CAD build for the part. Positions are in the model's coordinates, mm. Face numbers are marked on the shaded views. A direction names the side the tool comes from. Coordinates: 2 decimals unless noted, no trailing zeros. Write each loop counter-clockwise with the first axis right and the second up, starting at its lowest first coordinate (ties: lowest second). Pieces come first, ordered by that corner, then holes. Notation, with made-up numbers: (49, 53) - (96, 53) arc R34 cw to (96, 87) - close; hole circle Ø10 at (12, 26). An arc over 180 degrees is marked (long way). One line per question, with ' | ' between items. Start each with the question number.
1. Band-saw the part on C-C, the plane x = 85. Write the cut outline in (y, z).
2. Probe line 1 (X direction, y = -0.5, z = 56.5); line 2 (Z direction, x = 64, y = 27); line 3 (X direction, y = -10, z = 79). List the from-to ranges inside material, lowest first.
3. Two-plate mould, pull along X, no slides. Class the marked faces 1, 2 and 3: +X half, -X half, draft (parallel to the pull), parting line (faces both ways), or undercut.
4. Which spindle directions (+Z, -Z, +X, -X, +Y, -Y) get a long thin tool onto all of the face, cutting with end or side? Do the marked faces 4, 5 and 6. Say none if no direction does.
5. Band-saw the part on A-A, the plane y = 27. Write the cut outline in (x, z).
6. Flat gauge pins, fed straight in: P1, Ø10, axis at y = 30, z = 84.5, coming from the -X side; P2, Ø5, axis at y = -5.5, z = 50, coming from the +X side; P3, Ø4, axis at x = 78, y = 21, coming from the -Z side; P4, Ø3, axis at x = 39.5, y = 28, coming from the +Z side. Where does each tip first touch, or does it go through?
7. Band-saw the part on B-B, the plane y = -12. Write the cut outline in (x, z).
from build123d import *

# Parameters (mm, degrees)
F0_R      = 30
F1_DEPTH  = 20
F2_R      = 21.9
F3_DEPTH  = 5
F4_SIZE   = 2
F5_DEPTH  = 42
F6_R      = 21.9
F6_R_2    = 19.9
F7_DEPTH  = 3
F9_DEPTH  = 74.3
F11_R     = 4
F12_DEPTH = 25


with BuildPart() as f1:
    # F0 (on Front) → F1 (new body)
    with BuildSketch(Plane.XZ):
        with Locations((61.7417618632, 67.357480526)):
            Circle(F0_R)
    extrude(amount=F1_DEPTH)

    # F2 (on face) → F3 (join)
    with BuildSketch(Plane(origin=(0, 0, 0), x_dir=(-1, 0, 0), z_dir=(0, 1, 0))):
        with Locations((-61.7417618632, 67.357480526)):
            Circle(F2_R)
    extrude(amount=F3_DEPTH)

    # F4
    f4_edges = [f1.edges().sort_by_distance(p)[0] for p in [
        (83.641762, 5, 67.357481),
    ]]
    chamfer(f4_edges, length=F4_SIZE)

    # F5 (add): a face of the model
    f5_faces = [f1.faces().sort_by_distance(p)[0] for p in [
        (61.7417618632, 5, 67.357480526),
    ]]
    extrude(f5_faces, amount=F5_DEPTH)

    # F6 (on face) → F7 (join)
    with BuildSketch(Plane(origin=(0, 47, 0), x_dir=(-1, 0, 0), z_dir=(0, 1, 0))):
        with Locations((-61.7417618632, 67.357480526)):
            Circle(F6_R)
        with Locations((-61.7417618632, 67.357480526)):
            Circle(F6_R_2, mode=Mode.SUBTRACT)
        with Locations((-61.7417618632, 67.357480526)):
            Circle(F6_R_2)
    extrude(amount=F7_DEPTH)

    # F8 (on face) → F9 (cut)
    with BuildSketch(Plane(origin=(0, 50, 0), x_dir=(-1, 0, 0), z_dir=(0, 1, 0))):
        with BuildLine():
            Line((-79.7417618632, 63.357480526), (-76.198594158, 63.357480526))
            ThreePointArc((-76.198594158, 63.357480526), (-46.7417618632, 67.357480526), (-76.198594158, 71.357480526))
            Line((-76.198594158, 71.357480526), (-79.7417618632, 71.357480526))
            Line((-79.7417618632, 71.357480526), (-79.7417618632, 67.357480526))
            Line((-79.7417618632, 67.357480526), (-79.7417618632, 63.357480526))
        make_face()
    extrude(amount=-F9_DEPTH, mode=Mode.SUBTRACT)

    # F11 (on offset) → F12 (cut)
    with BuildSketch(Plane.XY.offset(100)):
        with Locations((62.0413188264, -9.8582830757)):
            Circle(F11_R)
    extrude(amount=-F12_DEPTH, mode=Mode.SUBTRACT)


solid = f1.part
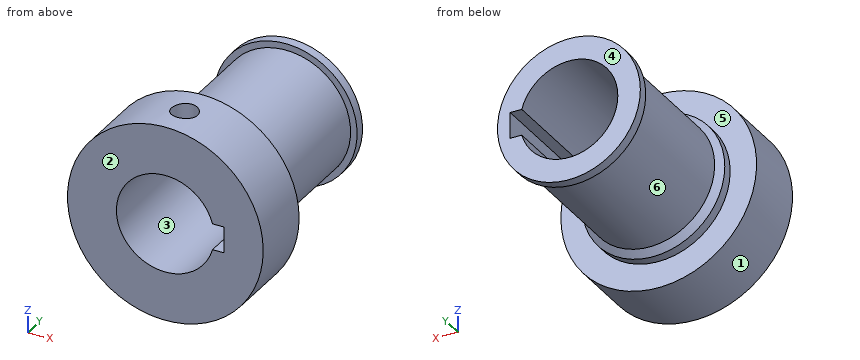
Filled in:
1) outline: (-20, 48.41) - (0, 48.41) - (0, 86.31) - (-20, 86.31) - close
2) line 1: x = 33.78 to 51.39, 72.09 to 89.71 | line 2: z = 47.59 to 52.53, 82.19 to 87.13 | line 3: x = 34.09 to 52.28, 71.2 to 89.39
3) face 1: parting line | face 2: draft | face 3: undercut
4) face 4: +Z, -Z, +X, -X, +Y | face 5: +Y | face 6: none
5) outline: circle Ø39.8 at (61.74, 67.36); hole (76.2, 63.36) - (79.74, 63.36) - (79.74, 71.36) - (76.2, 71.36) arc R15 ccw (long way) to start
6) P1: stops at x = 45.98 | P2: stops at x = 87.8 | P3: stops at z = 53.48 | P4: passes through
7) outline: (58.66, 82.04) - (58.66, 97.2) arc R30 ccw (long way) to (65.42, 97.13) - (65.42, 81.9) arc R15 cw to (76.2, 71.36) - (79.74, 71.36) - (79.74, 63.36) - (76.2, 63.36) arc R15 cw (long way) to start
